Input: part model. Units: mm. Frame: model coordinates. A direction names the side the tool comes from. Round coordinates to 2 decimals unless told otherwise and drop trailing zeros. Order: outer loops, then holes, each group sorted by start corner. A loop starts at its lowest first (then second) coordinate and runs counter-clockwise, first axis right, second up. Notation, with made-up numbers: (-23.5, 86.5) -> (9.5, 86.5) arc R23 cw to (9.5, 121.5) -> close; hole circle Ø1 at (83, 2). An arc over 180 degrees is marked (long way). Use a Markdown table: item, result.
from build123d import *

# Parameters (mm, degrees)
SKETCH1_W            = 177.8
SKETCH1_H            = 152.4
SKETCH1_R            = 3.3782
SKETCH1_R_2          = 2.667
BASE_FLANGE1_DEPTH   = 3.175
CHAMFER2_SIZE        = 3.175
SKETCH7_W            = 50.8
SKETCH7_H            = 25.4
CUT_EXTRUDE2_DEPTH   = 235.197951795
EDGE_FLANGE1_START   = 65.0875
EDGE_FLANGE1_DEPTH   = 47.625
EDGE_FLANGE1_2_DEPTH = 1.5875
EDGE_FLANGE1_START_2 = 111.125
EDGE_FLANGE1_3_DEPTH = 1.5875
EDGE_FLANGE1_START_3 = 66.675
EDGE_FLANGE1_4_DEPTH = 44.45
SKETCH11_W           = 1.5875
SKETCH11_H           = 6.50708023
CUT_EXTRUDE3_DEPTH   = 236.219607319
CHAMFER3_SIZE        = 3.175
SKETCH12_R           = 15.875
CUT_EXTRUDE4_DEPTH   = 236.219607319


# Read off the part's stored shape, not the designer's step: Edge-Flange1
# Sheet-metal steps are written as plain solids
with BuildPart() as part:
    # Sketch1 → Base-Flange1 (new body)
    with BuildSketch(Plane(origin=(0, 0, 0), x_dir=(1, 0, 0), z_dir=(0, 1, 0))):
        with Locations((88.9, 76.2)):
            Rectangle(SKETCH1_W, SKETCH1_H)
        with Locations(Location((38.1, 139.7, 0), (0, 0, 270))):
            Circle(SKETCH1_R, mode=Mode.SUBTRACT)
        with Locations(Location((139.7, 139.7, 0), (0, 0, 90))):
            Circle(SKETCH1_R, mode=Mode.SUBTRACT)
        with Locations(Location((12.7, 12.7, 0), (0, 0, 270))):
            Circle(SKETCH1_R_2, mode=Mode.SUBTRACT)
        with Locations(Location((165.1, 12.7, 0), (0, 0, 90))):
            Circle(SKETCH1_R_2, mode=Mode.SUBTRACT)
        with Locations(Location((63.5, 12.7, 0), (0, 0, 270))):
            Circle(SKETCH1_R_2, mode=Mode.SUBTRACT)
        with Locations(Location((114.3, 12.7, 0), (0, 0, 90))):
            Circle(SKETCH1_R_2, mode=Mode.SUBTRACT)
    extrude(amount=-BASE_FLANGE1_DEPTH)

    # Chamfer2
    chamfer2_edges = [part.edges().sort_by_distance(p)[0] for p in [
        (0, -1.5875, -152.4),
        (177.8, -1.5875, -152.4),
        (177.8, -1.5875, 0),
        (0, -1.5875, 0),
    ]]
    chamfer(chamfer2_edges, length=CHAMFER2_SIZE)

    # Sketch7 → Cut-Extrude2 (cut, through all)
    with BuildSketch(Plane(origin=(0, 0, 0), x_dir=(1, 0, 0), z_dir=(0, 1, 0))):
        with Locations((88.9, 65.0875)):
            Rectangle(SKETCH7_W, SKETCH7_H)
    extrude(amount=-CUT_EXTRUDE2_DEPTH, mode=Mode.SUBTRACT)

    # Edge-Flange1 outline → Edge-Flange1 (cut)
    with BuildSketch(Plane.YZ.offset(EDGE_FLANGE1_START)):
        with BuildLine():
            ThreePointArc((0, -51.958047831), (-2.301064967, -50.217550427), (-3.175, -47.46791977))
            Line((-3.175, -47.46791977), (-3.175, -52.3875))
            Line((-3.175, -52.3875), (0, -52.3875))
            Line((0, -52.3875), (0, -51.958047831))
        make_face()
    extrude(amount=EDGE_FLANGE1_DEPTH, mode=Mode.SUBTRACT)

    # Edge-Flange1 2 outline → Edge-Flange1 2 (cut)
    with BuildSketch(Plane.YZ.offset(EDGE_FLANGE1_START)):
        with BuildLine():
            Line((0, -45.88041977), (-3.175, -45.88041977))
            Line((-3.175, -45.88041977), (-3.175, -47.46791977))
            ThreePointArc((-3.175, -47.46791977), (-2.301064967, -50.217550427), (0, -51.958047831))
            Line((0, -51.958047831), (0, -45.88041977))
        make_face()
    extrude(amount=EDGE_FLANGE1_2_DEPTH, mode=Mode.SUBTRACT)

    # Edge-Flange1 3 outline → Edge-Flange1 3 (cut)
    with BuildSketch(Plane.YZ.offset(EDGE_FLANGE1_START_2)):
        with BuildLine():
            Line((0, -45.88041977), (-3.175, -45.88041977))
            Line((-3.175, -45.88041977), (-3.175, -47.46791977))
            ThreePointArc((-3.175, -47.46791977), (-2.301064967, -50.217550427), (0, -51.958047831))
            Line((0, -51.958047831), (0, -45.88041977))
        make_face()
    extrude(amount=EDGE_FLANGE1_3_DEPTH, mode=Mode.SUBTRACT)

    # Edge-Flange1 4 outline → Edge-Flange1 4 (add)
    with BuildSketch(Plane.YZ.offset(EDGE_FLANGE1_START_3)):
        with BuildLine():
            ThreePointArc((1.725859742, -49.049378854), (0.515000545, -48.638347543), (0, -47.46791977))
            Line((0, -47.46791977), (0, -51.958047831))
            ThreePointArc((0, -51.958047831), (0.987663955, -52.19249414), (2.002579225, -52.21229702))
            Line((2.002579225, -52.21229702), (22.128345332, -50.451520641))
            Line((22.128345332, -50.451520641), (21.851625848, -47.288602474))
            Line((21.851625848, -47.288602474), (1.725859742, -49.049378854))
        make_face()
    extrude(amount=EDGE_FLANGE1_4_DEPTH)

    # Sketch11 → Cut-Extrude3 (cut, through all)
    with BuildSketch(Plane(origin=(0, 0, 0), x_dir=(1, 0, 0), z_dir=(0, 1, 0))):
        with Locations((64.29375, 49.133959885)):
            Rectangle(SKETCH11_W, SKETCH11_H)
        with Locations((113.50625, 49.133959885)):
            Rectangle(SKETCH11_W, SKETCH11_H)
    extrude(amount=-CUT_EXTRUDE3_DEPTH, mode=Mode.SUBTRACT)

    # Chamfer3
    chamfer3_edges = [part.edges().sort_by_distance(p)[0] for p in [
        (111.125, 21.98998559, -48.870061558),
        (66.675, 21.98998559, -48.870061558),
    ]]
    chamfer(chamfer3_edges, length=CHAMFER3_SIZE)

    # Sketch12 → Cut-Extrude4 (cut, through all)
    with BuildSketch(Plane(origin=(0, 0, 0), x_dir=(1, 0, 0), z_dir=(0, 1, 0))):
        with Locations(Location((88.9, 108.74375, 0), (0, 0, 270))):
            Circle(SKETCH12_R)
        with Locations(Location((146.05, 108.74375, 0), (0, 0, 270))):
            Circle(SKETCH12_R)
        with Locations(Location((31.75, 108.74375, 0), (0, 0, 270))):
            Circle(SKETCH12_R)
    extrude(amount=-CUT_EXTRUDE4_DEPTH, mode=Mode.SUBTRACT)


solid = part.part
1) Cut plane D-D on x = 101. Return loops of the section in (y, z) (1 decimal).
Results found:
| item | result |
|---|---|
| outline | (-3.2, -152.4) -> (0, -152.4) -> (0, -119) -> (-3.2, -119) -> close; (-3.2, -98.5) -> (0, -98.5) -> (0, -77.8) -> (-3.2, -77.8) -> close; (-3.2, -47.5) arc R4.8 ccw to (2, -52.2) -> (22.1, -50.5) -> (21.9, -47.3) -> (1.7, -49) arc R1.6 cw to (0, -47.5) -> (0, 0) -> (-3.2, 0) -> close |
2) Cut plane B-B on z = -139.7. Return loops of the section in (x, y) (3 decimals).
Results found:
| item | result |
|---|---|
| outline | (0, -3.175) -> (34.722, -3.175) -> (34.722, 0) -> (0, 0) -> close; (41.478, -3.175) -> (136.322, -3.175) -> (136.322, 0) -> (41.478, 0) -> close; (143.078, -3.175) -> (177.8, -3.175) -> (177.8, 0) -> (143.078, 0) -> close |
3) Set-up query: faces 4 (the flat face through (66.675, 8, -50)), 5 (the flat face through (88.589, 11.925, -51.344)). Return all of +Z, -Z, +X, -X, +Y, -Y with unobstructed straight access to the full face (end or side cutting, diameter ignored); none if empty.
Results found:
| item | result |
|---|---|
| face 4 | +Y, -Y |
| face 5 | -Z, +X, -X, +Y |
4) Cut plane C-C on z = -12.7. Return loops of the section in (x, y) (3 decimals), and give its area (3 significant figures).
Results found:
| item | result |
|---|---|
| outline | (0, -3.175) -> (10.033, -3.175) -> (10.033, 0) -> (0, 0) -> close; (15.367, -3.175) -> (60.833, -3.175) -> (60.833, 0) -> (15.367, 0) -> close; (66.167, -3.175) -> (111.633, -3.175) -> (111.633, 0) -> (66.167, 0) -> close; (116.967, -3.175) -> (162.433, -3.175) -> (162.433, 0) -> (116.967, 0) -> close; (167.767, -3.175) -> (177.8, -3.175) -> (177.8, 0) -> (167.767, 0) -> close |
| area | 497 mm² |
5) Pull-direction query (Z, two-part tool) for faces 1 (the flat face through (107, -3.175, -94)), 2 (the flat face through (88.589, 11.93, -48.157)), 3 (the cylindrical face through (79.24, -1.57, -121.34)); classes: +Z half, -Z half, draft (parallel to the pull), parting line (faces both ways), or undercut.
Results found:
| item | result |
|---|---|
| face 1 | draft |
| face 2 | +Z half |
| face 3 | undercut |
6) Cut plane A-A on x = 146.05. Return loops of the section in (y, z) (3 decimals).
Results found:
| item | result |
|---|---|
| outline | (-3.175, -152.4) -> (0, -152.4) -> (0, -124.619) -> (-3.175, -124.619) -> close; (-3.175, -92.869) -> (0, -92.869) -> (0, 0) -> (-3.175, 0) -> close |
7) Pin query (flat end, axial travel): pin 1 Ø1.5 at (x, y) = (72, 15.5) entering from -Z; pin 2 Ø6 at (x, z) = (93.5, -30.5) entering from +Y; pin 3 Ø3 at (y, z) = (10.5, -50.5) entering from -X (3 decimals). Return the tip coordinate at first contact, or that it passes through.
Results found:
| item | result |
|---|---|
| pin 1 | stops at z = -51.1 |
| pin 2 | stops at y = 0 |
| pin 3 | stops at x = 66.675 |
8) Line query: L1, parallel to X at y = -1.2, z = -12.7; L2, parallel to X at y = -2.1, z = -139.7; L3, parallel to X at y = -0.75, z = -123. Output: solid intervals per line, ascending. Write a range as [from, to].
Results found:
| item | result |
|---|---|
| L1 | x = [0, 10.03], [15.37, 60.83], [66.17, 111.63], [116.97, 162.43], [167.77, 177.8] |
| L2 | x = [0, 34.72], [41.48, 136.32], [143.08, 177.8] |
| L3 | x = [0, 24.77], [38.73, 81.92], [95.88, 139.07], [153.03, 177.8] |
